Can you work these out from the model? Positions are in its coordinate system, mm. Round coordinates to 2 decimals unless told otherwise and drop trailing zeros. Loops run counter-clockwise (first coordinate to the right, second up) from the corner with the lowest first, then second, coordinate; pieces in that order, holes last. Notation, with made-up numbers: (-30, -13) -> (26, -13) arc R18 ccw to (26, 19) -> close; hole circle Ø5 at (39.5, 8). An arc over 180 degrees is marked (long way). Write each question's results on one line, items separated by ' | '.
from build123d import *

# Parameters (mm, degrees)
BOSS_EXTRUDE1_DEPTH             = 1.5875
F_5_32_0_15625_DIAMETER_HOLE1_D = 3.96875


with BuildPart() as part:
    # Sketch1 → Boss-Extrude1 (new body)
    with BuildSketch(Plane(origin=(0, 0, 0), x_dir=(1, 0, 0), z_dir=(0, 1, 0))):
        with BuildLine():
            Line((-160.755952561, 205.005137025), (-166.848726493, 205.005137025))
            Line((-166.848726493, 205.005137025), (-166.848726493, 173.255137025))
            Line((-166.848726493, 173.255137025), (-198.598726493, 173.255137025))
            Line((-198.598726493, 173.255137025), (-198.598726493, -169.644862975))
            Line((-198.598726493, -169.644862975), (-166.848726493, -169.644862975))
            Line((-166.848726493, -169.644862975), (-166.848726493, -201.394862975))
            Line((-166.848726493, -201.394862975), (-160.498726493, -201.394862975))
            ThreePointArc((-160.498726493, -201.394862975), (-158.638854554, -196.904734914), (-154.148726493, -195.044862975))
            Line((-154.148726493, -195.044862975), (150.651273507, -195.044862975))
            ThreePointArc((150.651273507, -195.044862975), (155.141401567, -196.904734914), (157.001273507, -201.394862975))
            Line((157.001273507, -201.394862975), (163.351273507, -201.394862975))
            Line((163.351273507, -201.394862975), (163.351273507, -169.644862975))
            Line((163.351273507, -169.644862975), (195.101273507, -169.644862975))
            Line((195.101273507, -169.644862975), (195.101273507, 173.255137025))
            Line((195.101273507, 173.255137025), (163.351273507, 173.255137025))
            Line((163.351273507, 173.255137025), (163.351273507, 205.005137025))
            Line((163.351273507, 205.005137025), (157.258499575, 205.005137025))
            ThreePointArc((157.258499575, 205.005137025), (155.323287864, 200.333122668), (150.651273507, 198.397910957))
            Line((150.651273507, 198.397910957), (-154.148726493, 198.397910957))
            ThreePointArc((-154.148726493, 198.397910957), (-158.820740851, 200.333122668), (-160.755952561, 205.005137025))
        make_face()
    extrude(amount=BOSS_EXTRUDE1_DEPTH)

    # 5/32 (0.15625) Diameter Hole1 (through all)
    with Locations(Plane(origin=(0, 1.5875, 0), x_dir=(1, 0, 0), z_dir=(0, 1, 0))):
        with Locations((-195.423726493, 78.005137025), (-195.423726493, -74.394862975), (191.926273507, -74.394862975), (191.926273507, 78.005137025)):
            Hole(F_5_32_0_15625_DIAMETER_HOLE1_D / 2)


solid = part.part
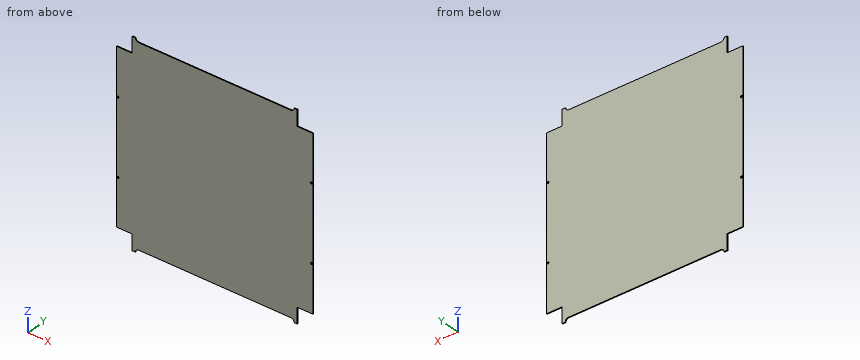
1. If we section it at B-B (x = 1): List the corners of the cut face in (y, z) for me.
Final values:
outline: (0, -198.4) -> (1.59, -198.4) -> (1.59, 195.04) -> (0, 195.04) -> close
2. Will these pins go through, and if not, where does the flat tip stop? pin 1 (2 mm diameter, centred on x = 50, z = -156.5, fed in from -Y); pin 2 (0.8 mm diameter, centred on x = 177.5, y = 0.5, fed in from -Z); pin 3 (0.8 mm diameter, centred on y = 1, z = 192.5, fed in from +X); pin 4 (2.5 mm diameter, centred on x = -195.42, z = -78.01, fed in from -Y).
Final values:
pin 1: y = 0 | pin 2: z = -173.26 | pin 3: x = 163.35 | pin 4: through
3. If we section it at A-A (y = 0.8): List the corners of the cut face in (x, z) for me, then the cut area to 3 significant figures.
Final values:
outline: (-198.6, -173.26) -> (-166.85, -173.26) -> (-166.85, -205.01) -> (-160.76, -205.01) arc R6.61 cw to (-154.15, -198.4) -> (150.65, -198.4) arc R6.61 cw to (157.26, -205.01) -> (163.35, -205.01) -> (163.35, -173.26) -> (195.1, -173.26) -> (195.1, 169.64) -> (163.35, 169.64) -> (163.35, 201.39) -> (157, 201.39) arc R6.35 cw to (150.65, 195.04) -> (-154.15, 195.04) arc R6.35 cw to (-160.5, 201.39) -> (-166.85, 201.39) -> (-166.85, 169.64) -> (-198.6, 169.64) -> close; hole circle Ø3.97 at (-195.42, -78.01); hole circle Ø3.97 at (-195.42, 74.39); hole circle Ø3.97 at (191.93, -78.01); hole circle Ø3.97 at (191.93, 74.39) | area: 152,000 mm2
4. Please list where these lines run through material, in increasing order: line 1 (Z direction, x = -60, y = 0.45); line 2 (Z direction, x = 163.5, y = 1.3); line 3 (X direction, y = 0.1, z = -186). Write a range as from..to.
Final values:
line 1: -198.4..195.04 | line 2: -173.26..169.64 | line 3: -166.85..163.35
